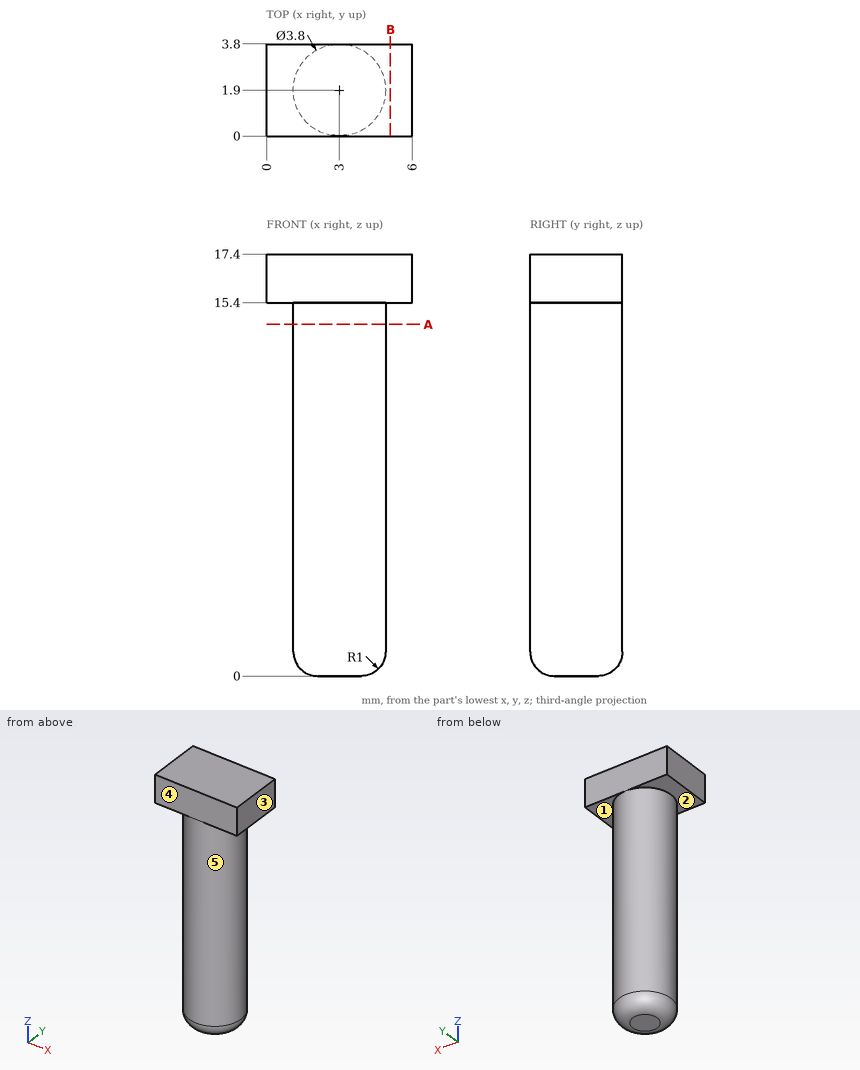
The drawing under review shows one solid part. Ordinate dimensions are in mm from its lowest x, y, z. A direction names the side the tool comes from. Round coordinates to 2 decimals unless told otherwise and drop trailing zeros. Loops run counter-clockwise (first coordinate to the right, second up) from the corner with the lowest first, then second, coordinate; pieces in that order, holes last. Notation, with made-up numbers: (60, 52.25) - (80, 52.25) arc R21 ccw to (80, 84.25) - close; hole circle Ø6 at (-0.75, 33). An arc over 180 degrees is marked (long way). Use a Markdown table: item, result. Add a question column.
Q1. For probe 1 along Z at (x, y) = (0.85, 0.3); probe 2 along X at (y, z) = (1.8, 13.25); probe 3 along Z at (x, y) = (3.25, 2.85), list the stretches that pass through material, from the lowest coordinate up.
Q2. Add section A-A (z = 14.5). State the section outline as (x, y) points, plus the area to 3 significant figures.
Q3. Machinability: for the marked faces 1, 2, 3, 4 and 5, which of the approach directions +Z, -Z, +X, -X, +Y, -Y give a long, thin tool a straight path to every point of the face, cutting with its end or side? Answer none if there is none.
Q4. Add section B-B (x = 5.1). State the section outline as (y, z) points, plus the area to 3 significant figures.
Worked answers:
| question | item | result |
|---|---|---|
| 1 | probe 1 | 15.4 to 17.4 |
| 1 | probe 2 | 1.1 to 4.9 |
| 1 | probe 3 | 0 to 17.4 |
| 2 | outline | circle Ø3.8 at (3, 1.9) |
| 2 | area | 11.3 mm² |
| 3 | face 1 | -Z, +X |
| 3 | face 2 | -Z, -X |
| 3 | face 3 | +Z, -Z, +X, +Y, -Y |
| 3 | face 4 | +Z, -Z, +X, -X, -Y |
| 3 | face 5 | -Z |
| 4 | outline | (0, 15.4) - (3.8, 15.4) - (3.8, 17.4) - (0, 17.4) - close |
| 4 | area | 7.60 mm² |
